Can you work these out from the model? Positions are in its coordinate system, mm. A direction names the side the tool comes from. Coordinates: 2 decimals unless noted, no trailing zeros. Order: outer loops, then holes, each group sorted by start corner. A loop starts at its lowest first (then second) coordinate and runs counter-clockwise, first axis right, second up. Notation, with made-up numbers: (29, 84) -> (47, 84) arc R12 cw to (47, 104) -> close; hole circle Ø6 at (2.5, -29). An arc over 180 degrees is marked (long way). Return JSON: item names as keys, results as strings. Group by question number.
1) For pin 1 (1.5 mm diameter, centred on x = 47, y = 23, fed in from +Z); pin 2 (3 mm diameter, centred on x = 11, z = 16.5, fed in from +Y); pin 3 (8 mm diameter, centred on y = 22, z = -4, fed in from -X); pin 4 (4 mm diameter, centred on x = 31, z = 10.5, fed in from +Y), each with a flat end and sliding along its axis, tell me the tip position at first contact or that it passes through.
2) If we section it at A-A, the plane z = -12: Please give me the cut outline in (x, y).
3) If we section it at B-B, the plane x = 36: Please give me the cut outline in (y, z), then the cut area to 3 significant figures.
4) Thinking about a two-plate mould opening in Z: for faces 1 (the flat face through (6, 21, -10)), 2 (the flat face through (85, 20, 5)), 3 (the cylindrical face through (25.436, 48.535, 9.525)), 4 (the cylindrical face through (10.826, 2.535, 4.605)), which applies, +Z half, -Z half, draft (parallel to the pull), parting line (faces both ways), or undercut?
5) For faces 5 (the flat face through (43, 22, -10)), 6 (the flat face through (-4, 6, 18)), 7 (the flat face through (17.05, 3, 10)), 8 (the flat face through (68, 5, 10)), which set-ups out of +Z, -Z, +X, -X, +Y, -Y let a thin tool reach every point of the face, with its end or its side?
6) If I drill on probe 1 along X at (y, z) = (32, 9); probe 2 along Y at (x, z) = (88, 17.3); probe 3 along Y at (x, z) = (64, 16), over which ranges is the centre line in solid material (lowest first)? Write a range as from..to.
from build123d import *

# Parameters (mm, degrees)
BOSS_EXTRUDE3_DEPTH  = 20
SKETCH4_W            = 85
SKETCH4_H            = 41
BOSS_EXTRUDE4_DEPTH  = 10
SKETCH5_R            = 2.5
CUT_EXTRUDE1_DEPTH   = 5
CUT_EXTRUDE2_START   = -5
SKETCH6_R            = 2.5
CUT_EXTRUDE2_DEPTH   = 5
FILLET2_R            = 1
SKETCH7_R            = 1.5
CUT_EXTRUDE3_DEPTH   = 5
CUT_EXTRUDE4_DEPTH   = 10
FILLET3_R            = 1
SKETCH10_W           = 50
SKETCH10_H           = 50
BOSS_EXTRUDE7_DEPTH  = 5
SKETCH9_W            = 50
SKETCH9_H            = 50
BOSS_EXTRUDE8_DEPTH  = 5
SKETCH11_R           = 0.75
CUT_EXTRUDE5_DEPTH   = 5
CHAMFER1_SIZE        = 2
CHAMFER2_SIZE        = 3
SKETCH15_W           = 6
SKETCH15_H           = 6
SKETCH15_R           = 1.5
BOSS_EXTRUDE11_DEPTH = 5
LPATTERN1_COUNT      = 2
LPATTERN1_PITCH      = 35
LPATTERN1_COUNT_DIR2 = 2
LPATTERN1_PITCH_DIR2 = 91
FILLET5_R            = 1
SKETCH16_R           = 2.5
BOSS_EXTRUDE12_DEPTH = 10
SKETCH17_R           = 1.5
CUT_EXTRUDE8_DEPTH   = 5


with BuildPart() as part:
    # Sketch3 → Boss-Extrude3 (new body)
    with BuildSketch(Plane.XY):
        Polygon((5, 36), (5, 5), (17.05, 5), (17.05, 0), (0, 0), (0, 41), (5, 41), (80, 41), (85, 41), (85, 0), (56.95, 0), (56.95, 5), (80, 5), (80, 36), align=None)
    extrude(amount=BOSS_EXTRUDE3_DEPTH)

    # Sketch4 → Boss-Extrude4 (add)
    with BuildSketch(Plane(origin=(0, 0, 0), x_dir=(-1, 0, 0), z_dir=(0, 0, -1))):
        with Locations((-42.5, 20.5)):
            Rectangle(SKETCH4_W, SKETCH4_H)
    extrude(amount=BOSS_EXTRUDE4_DEPTH)

    # Sketch5 → Cut-Extrude1 (cut)
    with BuildSketch(Plane(origin=(0, 5, 0), x_dir=(1, 0, 0), z_dir=(0, 1, 0))):
        with Locations(Location((71.95, -10, 0), (0, 0, 270))):
            Circle(SKETCH5_R)
    extrude(amount=-CUT_EXTRUDE1_DEPTH, mode=Mode.SUBTRACT)

    # Sketch6 → Cut-Extrude2 (cut)
    with BuildSketch(Plane.XZ.offset(-36).offset(CUT_EXTRUDE2_START)):
        with Locations(Location((71.95, 10, 0), (0, 0, 90))):
            Circle(SKETCH6_R)
    extrude(amount=CUT_EXTRUDE2_DEPTH, mode=Mode.SUBTRACT)

    # Fillet2
    fillet2_edges = [part.edges().sort_by_distance(p)[0] for p in [
        (71.95, 5, 7.5),
        (71.95, 36, 7.5),
    ]]
    fillet(fillet2_edges, radius=FILLET2_R)

    # Sketch7 → Cut-Extrude3 (cut)
    with BuildSketch(Plane(origin=(0, 5, 0), x_dir=(1, 0, 0), z_dir=(0, 1, 0))):
        with Locations(Location((12.29, -4.93, 0), (0, 0, 270))):
            Circle(SKETCH7_R)
        with Locations(Location((12.29, -14.78, 0), (0, 0, 270))):
            Circle(SKETCH7_R)
    cut_extrude3 = extrude(amount=-CUT_EXTRUDE3_DEPTH, mode=Mode.SUBTRACT)

    # Mirror1: Cut-Extrude3 across plane
    add(cut_extrude3.mirror(Plane(origin=(37, 0, 0), x_dir=(0, 0, 1), z_dir=(1, 0, 0))), mode=Mode.SUBTRACT)

    # Sketch8 → Cut-Extrude4 (cut)
    with BuildSketch(Plane.XY):
        with BuildLine():
            Line((13, 27.5), (13, 12.5))
            ThreePointArc((13, 12.5), (10, 9.5), (7, 12.5))
            Line((7, 12.5), (7, 27.5))
            ThreePointArc((7, 27.5), (10, 30.5), (13, 27.5))
        make_face()
    extrude(amount=-CUT_EXTRUDE4_DEPTH, mode=Mode.SUBTRACT)

    # Fillet3
    fillet3_edges = [part.edges().sort_by_distance(p)[0] for p in [
        (10, 30.5, 0),
        (7, 20, 0),
        (10, 9.5, 0),
        (13, 20, 0),
    ]]
    fillet(fillet3_edges, radius=FILLET3_R)

    # Sketch10 → Boss-Extrude7 (add)
    with BuildSketch(Plane(origin=(0, 0, -10), x_dir=(-1, 0, 0), z_dir=(0, 0, -1))):
        with Locations((-42.5, 20.5)):
            Rectangle(SKETCH10_W, SKETCH10_H)
    extrude(amount=-BOSS_EXTRUDE7_DEPTH)

    # Sketch9 → Boss-Extrude8 (add)
    with BuildSketch(Plane(origin=(0, 0, -10), x_dir=(-1, 0, 0), z_dir=(0, 0, -1))):
        with Locations((-42.5, 20.5)):
            Rectangle(SKETCH9_W, SKETCH9_H)
        with BuildLine():
            Line((-59.2, 24.3), (-48.011787453, 24.5))
            ThreePointArc((-48.011787453, 24.5), (-46.919880362, 24.919880362), (-46.5, 26.011787453))
            Line((-46.5, 26.011787453), (-46.3, 37.2))
            ThreePointArc((-46.3, 37.2), (-42.5, 41), (-38.7, 37.2))
            Line((-38.7, 37.2), (-38.5, 26.011787453))
            ThreePointArc((-38.5, 26.011787453), (-38.080119638, 24.919880362), (-36.988212547, 24.5))
            Line((-36.988212547, 24.5), (-25.8, 24.3))
            ThreePointArc((-25.8, 24.3), (-22, 20.5), (-25.8, 16.7))
            Line((-25.8, 16.7), (-36.988212547, 16.5))
            ThreePointArc((-36.988212547, 16.5), (-38.080119638, 16.080119638), (-38.5, 14.988212547))
            Line((-38.5, 14.988212547), (-38.7, 3.8))
            ThreePointArc((-38.7, 3.8), (-42.5, 0), (-46.3, 3.8))
            Line((-46.3, 3.8), (-46.5, 14.988212547))
            ThreePointArc((-46.5, 14.988212547), (-46.919880362, 16.080119638), (-48.011787453, 16.5))
            Line((-48.011787453, 16.5), (-59.2, 16.7))
            ThreePointArc((-59.2, 16.7), (-63, 20.5), (-59.2, 24.3))
        make_face(mode=Mode.SUBTRACT)
    extrude(amount=BOSS_EXTRUDE8_DEPTH)

    # Sketch11 → Cut-Extrude5 (cut)
    with BuildSketch(Plane(origin=(0, 0, -10), x_dir=(-1, 0, 0), z_dir=(0, 0, -1))):
        with Locations((-59, 20.5)):
            Circle(SKETCH11_R)
        with Locations(Location((-26, 20.5, 0), (0, 0, 180))):
            Circle(SKETCH11_R)
    extrude(amount=-CUT_EXTRUDE5_DEPTH, mode=Mode.SUBTRACT)

    # Chamfer1
    chamfer1_edges = [part.edges().sort_by_distance(p)[0] for p in [
        (42.5, 45.5, -5),
        (42.5, -4.5, -5),
        (67.5, 20.5, -15),
        (42.5, -4.5, -15),
        (17.5, 20.5, -15),
        (42.5, 45.5, -15),
    ]]
    chamfer(chamfer1_edges, length=CHAMFER1_SIZE)

    # Chamfer2
    chamfer2_edges = [part.edges().sort_by_distance(p)[0] for p in [
        (17.5, 20.5, -10),
        (67.5, 20.5, -10),
    ]]
    chamfer(chamfer2_edges, length=CHAMFER2_SIZE - 0.0001)  # a hair under: the kernel refuses the full size

    # Sketch15 → Boss-Extrude11 (add)
    with BuildSketch(Plane.XY.offset(20)):
        with Locations((-3, 38)):
            Rectangle(SKETCH15_W, SKETCH15_H)
        with Locations((-3, 38)):
            Circle(SKETCH15_R, mode=Mode.SUBTRACT)
    boss_extrude11 = extrude(amount=-BOSS_EXTRUDE11_DEPTH)

    # LPattern1: Boss-Extrude11 2 × 2
    with Locations(*[(j * LPATTERN1_PITCH_DIR2, -i * LPATTERN1_PITCH, 0) for i in range(LPATTERN1_COUNT) for j in range(LPATTERN1_COUNT_DIR2) if (i, j) != (0, 0)]):
        add(boss_extrude11)

    # Fillet5
    fillet5_edges = [part.edges().sort_by_distance(p)[0] for p in [
        (0, 38, 15),
        (0, 35, 17.5),
        (85, 38, 15),
        (85, 35, 17.5),
        (0, 3, 15),
        (0, 6, 17.5),
        (85, 3, 15),
        (85, 6, 17.5),
    ]]
    fillet(fillet5_edges, radius=FILLET5_R)

    # Sketch16 → Boss-Extrude12 (add)
    with BuildSketch(Plane(origin=(0, 41, 0), x_dir=(1, 0, 0), z_dir=(0, 1, 0))):
        with Locations(Location((26.900249723, -9.85, 0), (0, 0, 90))):
            Circle(SKETCH16_R)
    extrude(amount=BOSS_EXTRUDE12_DEPTH)

    # Sketch17 → Cut-Extrude8 (cut)
    with BuildSketch(Plane(origin=(0, 51, 0), x_dir=(1, 0, 0), z_dir=(0, 1, 0))):
        with Locations(Location((26.900249723, -9.85, 0), (0, 0, 270))):
            Circle(SKETCH17_R)
    extrude(amount=-CUT_EXTRUDE8_DEPTH, mode=Mode.SUBTRACT)


solid = part.part
Result sheet:
{
 "1": {"pin 1": "stops at z = 0", "pin 2": "stops at y = 41", "pin 3": "stops at x = 0", "pin 4": "stops at y = 51"},
 "2": {"outline": "(16.5, 0) -> (17.5, 0) -> (17.5, -4.5) -> (67.5, -4.5) -> (67.5, 0) -> (68.5, 0) -> (68.5, 41) -> (67.5, 41) -> (67.5, 45.5) -> (17.5, 45.5) -> (17.5, 41) -> (16.5, 41) -> close; hole (25.8, 16.7) -> (36.99, 16.5) arc R1.44 cw to (38.5, 14.99) -> (38.7, 3.8) arc R3.8 ccw to (46.3, 3.8) -> (46.5, 14.99) arc R1.44 cw to (48.01, 16.5) -> (59.2, 16.7) arc R3.8 ccw to (59.2, 24.3) -> (48.01, 24.5) arc R1.44 cw to (46.5, 26.01) -> (46.3, 37.2) arc R3.8 ccw to (38.7, 37.2) -> (38.5, 26.01) arc R1.44 cw to (36.99, 24.5) -> (25.8, 24.3) arc R3.8 ccw to start"},
 "3": {"outline": "(-4.5, -13) -> (-2.5, -15) -> (16.52, -15) -> (16.52, -10) -> (24.48, -10) -> (24.48, -15) -> (43.5, -15) -> (45.5, -13) -> (45.5, -7) -> (43.5, -5) -> (41, -5) -> (41, 20) -> (36, 20) -> (36, 0) -> (0, 0) -> (0, -5) -> (-2.5, -5) -> (-4.5, -7) -> close", "area": "757 mm2"},
 "4": {"face 1": "-Z half", "face 2": "draft", "face 3": "undercut", "face 4": "undercut"},
 "5": {"face 5": "-Z", "face 6": "+Z, -Z, -X", "face 7": "+Z, -Y", "face 8": "+Z"},
 "6": {"probe 1": "x = 0..5, 80..85", "probe 2": "y = 0..1.5, 4.5..6, 35..36.5, 39.5..41", "probe 3": "y = 0..5, 36..41"}
}
